Model file for the job. Use its own axes, mm. A direction names the side the tool comes from. Round coordinates to 2 decimals unless told otherwise and drop trailing zeros. Order: outer loops, then holes, each group sorted by start corner. A loop starts at its lowest first (then second) coordinate and runs counter-clockwise, first axis right, second up. Notation, with made-up numbers: (88, 17) -> (121, 17) arc R10 cw to (121, 29) -> close; hole circle Ø5 at (72, 20.25). An arc over 180 degrees is marked (long way). Put each result on its own line as item: value. Start each with the question number.
Q1. 3-axis set-ups, long thin cutter, end or side, ignore diameter. For faces 4 (the face through (122.5, -2, 2)), 5 (the face through (142, 20, 2)), 6 (the face through (120.9, 54, 2)): which of +Z, -Z, +X, -X, +Y, -Y reach the whole face in a straight line?
Q2. Probe L1, parallel to Y at x = 29, z = 1.15 (3 decimals); L2, parallel to Y at x = 120, z = 2.95 (3 decimals); L3, parallel to X at y = 42, z = 3.45. List the from-to ranges inside material, lowest first.
Q3. Cut at D-D, the plane x = 96.5. List the corners of the cut face in (y, z).
Q4. Pull direction X, two halves, no side cores. Call faces 1 (the face through (0, 46, 2)), 2 (the face through (142, 8.571, 2)), 3 (the face through (45.5, 82, 2)): released by +X, released by -X, zero draft, split by the parting line, or undercut.
Q5. Flat gauge pins, fed straight in: P1, Ø2, axis at x = 44, z = 2, coming from the -Y side; P2, Ø1.2, axis at x = 97, z = 2, coming from the +Y side; P3, Ø1, axis at y = 70, z = 2.5, coming from the +X side; P4, Ø11, axis at x = 45, y = 35, coming from the +Z side. Where does each tip first touch, or does it go through?
Q6. Cut at C-C, the plane z = 2.95. State how many separate pieces and enclosed holes the cut face has, and give its area (3 significant figures).
Q7. Cut at A-A, the plane x = 12. List the corners of the cut face in (y, z).
Q8. Cut at B-B, the plane y = 35. List the corners of the cut face in (x, z).
from build123d import *

# Parameters (mm, degrees)
SCHIZZO1_W                   = 140
SCHIZZO1_H                   = 80
SCHIZZO1_R                   = 6
SCHIZZO1_R_2                 = 3.9
ESTRUSIONE_ESTRUSIONE1_DEPTH = 4
SCHIZZO2_W                   = 7
SCHIZZO2_H                   = 4
ESTRUSIONE_ESTRUSIONE2_DEPTH = 4
RIPETIZIONE_A_L1_COUNT       = 10
RIPETIZIONE_A_L1_PITCH       = 14
SCHIZZO3_W                   = 4
SCHIZZO3_H                   = 5.714285714
ESTRUSIONE_ESTRUSIONE3_DEPTH = 4
RIPETIZIONE_A_L2_COUNT       = 7
RIPETIZIONE_A_L2_PITCH       = 11.428571429
SCHIZZO4_W                   = 4
SCHIZZO4_H                   = 6.25
TAGLIO_ESTRUSIONE1_DEPTH     = 167.757308685
RIPETIZIONE_A_L3_COUNT       = 4
RIPETIZIONE_A_L3_PITCH       = 12.5
SCHIZZO5_W                   = 4
SCHIZZO5_H                   = 6.25
TAGLIO_ESTRUSIONE2_DEPTH     = 167.757308685
RIPETIZIONE_A_L4_COUNT       = 4
RIPETIZIONE_A_L4_PITCH       = 12.5
SCHIZZO6_W                   = 4
SCHIZZO6_H                   = 4
TAGLIO_ESTRUSIONE3_DEPTH     = 167.757308685


with BuildPart() as part:
    # Schizzo1 → Estrusione-Estrusione1 (new body)
    with BuildSketch(Plane.XY):
        with Locations((70, 40)):
            Rectangle(SCHIZZO1_W, SCHIZZO1_H)
        with Locations((45, 35)):
            Circle(SCHIZZO1_R, mode=Mode.SUBTRACT)
        with Locations((95, 35)):
            Circle(SCHIZZO1_R, mode=Mode.SUBTRACT)
        with Locations((12, 12)):
            Circle(SCHIZZO1_R, mode=Mode.SUBTRACT)
        with Locations((70, 35)):
            Circle(SCHIZZO1_R_2, mode=Mode.SUBTRACT)
    extrude(amount=ESTRUSIONE_ESTRUSIONE1_DEPTH)

    # Schizzo2 → Estrusione-Estrusione2 (add)
    with BuildSketch(Plane.XY.offset(4)):
        with Locations((7, 82)):
            Rectangle(SCHIZZO2_W, SCHIZZO2_H)
        with Locations((7, -2)):
            Rectangle(SCHIZZO2_W, SCHIZZO2_H)
    estrusione_estrusione2 = extrude(amount=-ESTRUSIONE_ESTRUSIONE2_DEPTH)

    # Ripetizione a L1: Estrusione-Estrusione2 ×10
    with Locations(*[(i * RIPETIZIONE_A_L1_PITCH, 0, 0) for i in range(1, RIPETIZIONE_A_L1_COUNT)]):
        add(estrusione_estrusione2)

    # Schizzo3 → Estrusione-Estrusione3 (add)
    with BuildSketch(Plane.XY.offset(4)):
        with Locations((-2, 74.285714286)):
            Rectangle(SCHIZZO3_W, SCHIZZO3_H)
        with Locations((142, 74.285714286)):
            Rectangle(SCHIZZO3_W, SCHIZZO3_H)
    estrusione_estrusione3 = extrude(amount=-ESTRUSIONE_ESTRUSIONE3_DEPTH)

    # Ripetizione a L2: Estrusione-Estrusione3 ×7
    with Locations(*[(0, -i * RIPETIZIONE_A_L2_PITCH, 0) for i in range(1, RIPETIZIONE_A_L2_COUNT)]):
        add(estrusione_estrusione3)

    # Schizzo4 → Taglio-Estrusione1 (cut, through all)
    with BuildSketch(Plane.XY.offset(4)):
        with Locations((30, 53.75)):
            Rectangle(SCHIZZO4_W, SCHIZZO4_H)
    taglio_estrusione1 = extrude(amount=-TAGLIO_ESTRUSIONE1_DEPTH, mode=Mode.SUBTRACT)

    # Ripetizione a L3: Taglio-Estrusione1 ×4
    with Locations(*[(0, -i * RIPETIZIONE_A_L3_PITCH, 0) for i in range(1, RIPETIZIONE_A_L3_COUNT)]):
        add(taglio_estrusione1, mode=Mode.SUBTRACT)

    # Schizzo5 → Taglio-Estrusione2 (cut, through all)
    with BuildSketch(Plane(origin=(0, 0, 0), x_dir=(-1, 0, 0), z_dir=(0, 0, -1))):
        with Locations((-127, 53.75)):
            Rectangle(SCHIZZO5_W, SCHIZZO5_H)
        with Locations((-118.9, 53.75)):
            Rectangle(SCHIZZO5_W, SCHIZZO5_H)
    taglio_estrusione2 = extrude(amount=-TAGLIO_ESTRUSIONE2_DEPTH, mode=Mode.SUBTRACT)

    # Ripetizione a L4: Taglio-Estrusione2 ×4
    with Locations(*[(0, -i * RIPETIZIONE_A_L4_PITCH, 0) for i in range(1, RIPETIZIONE_A_L4_COUNT)]):
        add(taglio_estrusione2, mode=Mode.SUBTRACT)

    # Schizzo6 → Taglio-Estrusione3 (cut, through all)
    with BuildSketch(Plane(origin=(0, 0, 0), x_dir=(-1, 0, 0), z_dir=(0, 0, -1))):
        with Locations((-122.95, 15.634824405)):
            Rectangle(SCHIZZO6_W, SCHIZZO6_H)
        with Locations((-122.95, 24.894824405)):
            Rectangle(SCHIZZO6_W, SCHIZZO6_H)
    extrude(amount=-TAGLIO_ESTRUSIONE3_DEPTH, mode=Mode.SUBTRACT)


solid = part.part
Ans:
1. face 4: +Z, -Z, -Y
1. face 5: +Z, -Z, +X
1. face 6: +Z, -Z
2. L1: y = 0 to 13.125, 19.375 to 25.625, 31.875 to 38.125, 44.375 to 50.625, 56.875 to 80
2. L2: y = -4 to 13.125, 19.375 to 25.625, 31.875 to 38.125, 44.375 to 50.625, 56.875 to 84
2. L3: x = -4 to 28, 32 to 116.9, 120.9 to 125, 129 to 144
3. outline: (0, 0) -> (29.19, 0) -> (29.19, 4) -> (0, 4) -> close; (40.81, 0) -> (80, 0) -> (80, 4) -> (40.81, 4) -> close
4. face 1: released by -X
4. face 2: zero draft
4. face 3: undercut
5. P1: stops at y = 0
5. P2: stops at y = 80
5. P3: stops at x = 140
5. P4: passes through
6. separate pieces: 1
6. enclosed holes: 18
6. area: 11,400 mm^2
7. outline: (0, 0) -> (6, 0) -> (6, 4) -> (0, 4) -> close; (18, 0) -> (80, 0) -> (80, 4) -> (18, 4) -> close
8. outline: (0, 0) -> (39, 0) -> (39, 4) -> (0, 4) -> close; (51, 0) -> (66.1, 0) -> (66.1, 4) -> (51, 4) -> close; (73.9, 0) -> (89, 0) -> (89, 4) -> (73.9, 4) -> close; (101, 0) -> (140, 0) -> (140, 4) -> (101, 4) -> close
